Can you work these out from the drawing? Everything is in mm from the part's minimum corner. Coordinates: 2 decimals unless noted, no trailing zeros. Loops run counter-clockwise (first coordinate to the right, second up) from the corner with the lowest first, then second, coordinate; pieces in that order, holes last. Notation, with made-up numbers: (20, -25) - (54, -25) arc R21 cw to (54, 13) - close; hole circle Ø2 at (-21.5, 61.25). An arc over 180 degrees is marked (long way). One line per question, with ' | ' between items. Start each with the question number.
1. I want a section at B-B, the plane x = 55. Write out the boundary of the cut face in (y, z) (1 decimal), then the cut area to 3 significant figures.
2. Please list where these lines run through material, in increasing order: L1, parallel to X at y = 16.5, z = 23.5 (1 decimal); L2, parallel to Z at x = 89.5, y = 13 (1 decimal); L3, parallel to Z at x = 28, y = 7.5 (1 decimal). Write a range as [from, to].
3. I want a section at A-A, the plane y = 3.5. Write out the boundary of the cut face in (x, z) (1 decimal), then the cut area to 4 significant figures.
4. I want a section at C-C, the plane z = 44.5. Write out the boundary of the cut face in (x, y).
5. I'm going to push flat-ended pins straight in: P1, Ø4, axis at y = 14, z = 8.5, coming from the +X side (1 decimal); P2, Ø12, axis at y = 14.5, z = 13.5, coming from the +X side; P3, Ø2, axis at y = 18, z = 19, coming from the +X side (1 decimal); P4, Ø1.5, axis at x = 69.5, z = 14, coming from the +Y side. Where does each tip first touch, or does it pass through?
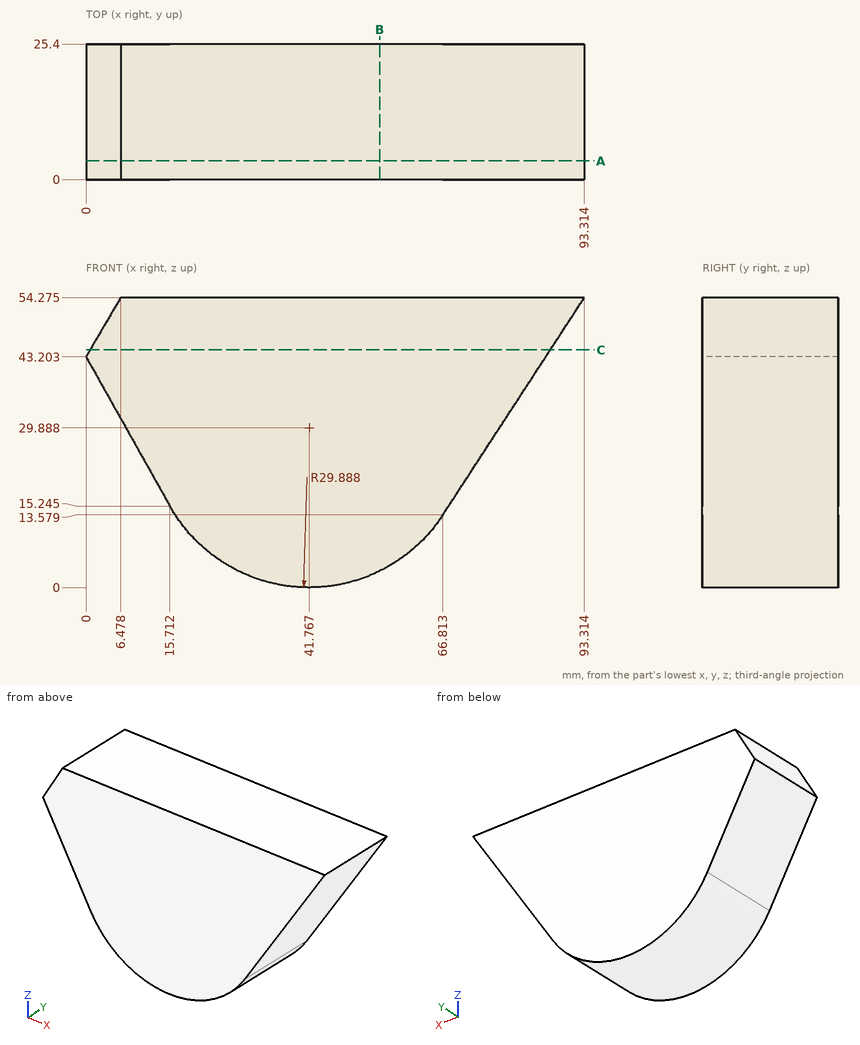
Results are:
1) outline: (0, 3.1) - (25.4, 3.1) - (25.4, 54.3) - (0, 54.3) - close | area: 1,300 mm2
2) L1: x = [11.1, 73.3] | L2: z = [48.4, 54.3] | L3: z = [3.4, 54.3]
3) outline: (0, 43.2) - (15.7, 15.2) arc R29.9 ccw to (66.8, 13.6) - (93.3, 54.3) - (6.5, 54.3) - close | area: 3,455 mm2
4) outline: (0.76, 0) - (86.95, 0) - (86.95, 25.4) - (0.76, 25.4) - close
5) P1: stops at x = 64.5 | P2: stops at x = 70.67 | P3: stops at x = 71 | P4: passes through
